Build history of the part. All positions in model axes, mm. A direction names the side the tool comes from. Coordinates: 2 decimals unless noted, no trailing zeros. Order: outer loops, then holes, each group sorted by start corner. A loop starts at its lowest first (then second) coordinate and runs counter-clockwise, first axis right, second up. Notation, with made-up numbers: (-6.75, -31) - (34.25, -31) arc R25 ccw to (34.25, -4) - close; hole circle Ø10 at (29, 86). An arc over 180 degrees is marked (long way). Write each question's results on one line, items separated by ' | '. Start each with the question number.
from build123d import *

# Parameters (mm, degrees)
EXTRUDE_1_DEPTH     = 70
CUT_EXTRUDE_1_DEPTH = 74.35529974
SKETCH_3_W          = 18.609369779
SKETCH_3_H          = 2.954088086
EXTRUDE_3_DEPTH     = 15.5
SKETCH_4_W          = 40
SKETCH_4_H          = 1
EXTRUDE_4_DEPTH     = 20
SKETCH_5_R          = 0.9
CUT_EXTRUDE_2_DEPTH = 72.281133549
SKETCH_6_W          = 3.6
SKETCH_6_H          = 3.5
SKETCH_7_R          = 1.25
CUT_EXTRUDE_3_DEPTH = 72.414284285


with BuildPart() as part:
    # ｽｹｯﾁ1 → ﾎﾞｽ - 押し出し1 (new body)
    with BuildSketch(Plane.XY):
        Polygon((-10, 0), (10, 0), (10, 3), (7.202154051, 9), (-7.202154051, 9), (-10, 3), align=None)
    extrude(amount=EXTRUDE_1_DEPTH)

    # ｽｹｯﾁ2 → ｶｯﾄ - 押し出し1 (cut, through all)
    with BuildSketch(Plane(origin=(10, 0, 0), x_dir=(0, 0, -1), z_dir=(1, 0, 0))):
        Polygon((-70, 3), (-67.202154051, 9), (-70, 9), align=None)
        Polygon((-2.797845949, 9), (0, 9), (0, 3), align=None)
    extrude(amount=-CUT_EXTRUDE_1_DEPTH, mode=Mode.SUBTRACT)

    # 面取り1
    # the kernel refuses this chamfer: 0.5 mm, written as the material it takes off along each edge
    with BuildSketch(Plane(origin=(-6.995420754, 8.697897404, 3.004579246), x_dir=(-0.8270486586180938, -0.5268881046463177, -0.19590671622030348), z_dir=(-0.41632572739388457, 0.8082980746110386, -0.41632572739387685))) as chamfer_1_piece_1:
        Polygon((-0.459173014, 0.228990916), (0.400884159, 0.228990916), (0.058288855, -0.457981831), align=None)
    extrude(amount=0.4579583, mode=Mode.SUBTRACT)
    with BuildSketch(Plane(origin=(-6.995420754, 8.697897404, 66.995420754), x_dir=(0.1959067162203077, 0.5268881046463173, -0.8270486586180933), z_dir=(-0.41632572739387774, 0.8082980746110393, 0.4163257273938825))) as chamfer_1_piece_2:
        Polygon((-0.400884159, -0.228990916), (0.459173014, -0.228990916), (-0.058288855, 0.457981831), align=None)
    extrude(amount=0.4579583, mode=Mode.SUBTRACT)
    with BuildSketch(Plane(origin=(6.995420754, 8.697897404, 3.004579246), x_dir=(0.8270486586180947, -0.5268881046463163, -0.1959067162203037), z_dir=(0.4163257273938817, 0.8082980746110384, -0.41632572739387985))) as chamfer_1_piece_3:
        Polygon((-0.459173014, -0.228990916), (0.400884159, -0.228990916), (0.058288855, 0.457981831), align=None)
    extrude(amount=0.4579583, mode=Mode.SUBTRACT)
    with BuildSketch(Plane(origin=(6.995420754, 8.697897404, 66.995420754), x_dir=(-0.19590671622030845, 0.5268881046463186, -0.8270486586180921), z_dir=(0.4163257273938828, 0.8082980746110372, 0.4163257273938814))) as chamfer_1_piece_4:
        Polygon((-0.400884159, 0.228990916), (0.459173014, 0.228990916), (-0.058288855, -0.457981831), align=None)
    extrude(amount=0.4579583, mode=Mode.SUBTRACT)
    with BuildSketch(Plane(origin=(10, -1.285841494, 70), x_dir=(0.02749587661058574, 0, -0.9996219169112968), z_dir=(0, 1, 0)), Plane(origin=(-10, 4.285841494, 70), x_dir=(-0.02749587661058574, 0, -0.9996219169112968), z_dir=(0, -1, 0))) as chamfer_1_piece_5:
        with BuildLine():
            Line((0.514336598, 0), (-0.028273577, 0.513558897))
            Line((-0.028273577, 0.513558897), (-0.038269797, 0.513283938))
            ThreePointArc((-0.038269797, 0.513283938), (-0.017064614, 0.256698915), (-0.009996219, -0.000274959))
            Line((-0.009996219, -0.000274959), (0.000274959, -0.009996219))
            ThreePointArc((0.000274959, -0.009996219), (0.257248832, -0.002927825), (0.514611556, -0.009996219))
            Line((0.514611556, -0.009996219), (0.514336598, 0))
        make_face()
    extrude(amount=5.571682988, mode=Mode.SUBTRACT)
    with BuildSketch(Plane(origin=(-7.202154051, 9, 1.505397137), x_dir=(-0.4413655645980917, -0.8973273864019796, 0), z_dir=(0, 0, 1))) as chamfer_1_piece_6:
        with BuildLine():
            Line((0.516979525, 0), (-0.237770334, 0.459056747))
            Line((-0.237770334, 0.459056747), (-0.246743608, 0.454643091))
            ThreePointArc((-0.246743608, 0.454643091), (-0.123037104, 0.227486173), (-0.008973274, -0.004413656))
            Line((-0.008973274, -0.004413656), (0.000207861, -0.009997839))
            ThreePointArc((0.000207861, -0.009997839), (0.25858594, -0.004626004), (0.517187386, -0.009997839))
            Line((0.517187386, -0.009997839), (0.516979525, 0))
        make_face()
    extrude(amount=66.989205725, mode=Mode.SUBTRACT)
    with BuildSketch(Plane(origin=(7.202154051, 9, 1.505397137), x_dir=(0.441365564598093, -0.897327386401979, 0), z_dir=(0, 0, 1))) as chamfer_1_piece_7:
        with BuildLine():
            Line((0.516979525, 0), (-0.237770334, -0.459056747))
            Line((-0.237770334, -0.459056747), (-0.246743608, -0.454643091))
            ThreePointArc((-0.246743608, -0.454643091), (-0.123037104, -0.227486173), (-0.008973274, 0.004413656))
            Line((-0.008973274, 0.004413656), (0.000207861, 0.009997839))
            ThreePointArc((0.000207861, 0.009997839), (0.25858594, 0.004626004), (0.517187386, 0.009997839))
            Line((0.517187386, 0.009997839), (0.516979525, 0))
        make_face()
    extrude(amount=66.989205725, mode=Mode.SUBTRACT)
    with BuildSketch(Plane(origin=(8.494602863, 9, 67.202154051), x_dir=(0, -0.8973273864019776, 0.4413655645980958), z_dir=(-1, 0, 0))) as chamfer_1_piece_8:
        with BuildLine():
            Line((0.516979525, 0), (-0.237770334, -0.459056747))
            Line((-0.237770334, -0.459056747), (-0.246743608, -0.454643091))
            ThreePointArc((-0.246743608, -0.454643091), (-0.123037104, -0.227486173), (-0.008973274, 0.004413656))
            Line((-0.008973274, 0.004413656), (0.000207861, 0.009997839))
            ThreePointArc((0.000207861, 0.009997839), (0.25858594, 0.004626004), (0.517187386, 0.009997839))
            Line((0.517187386, 0.009997839), (0.516979525, 0))
        make_face()
    extrude(amount=16.989205725, mode=Mode.SUBTRACT)
    with BuildSketch(Plane(origin=(6.700455124, 10.075896822, 66.700455124), x_dir=(0.18700008699946485, -0.3421923931836809, -0.920834042327616), z_dir=(0.38928162063502725, -0.83481712947899, 0.38928162063501803)), Plane(origin=(-10.501698928, 1.924103178, 70.501698928), x_dir=(-0.1870000869994657, -0.34219239318368055, -0.920834042327616), z_dir=(0.38928162063502697, 0.8348171294789901, -0.3892816206350181))) as chamfer_1_piece_9:
        with BuildLine():
            Line((0.515512576, 0), (-0.117174183, -0.502019349))
            Line((-0.117174183, -0.502019349), (-0.126965941, -0.499989208))
            ThreePointArc((-0.126965941, -0.499989208), (-0.062103739, -0.250280562), (-0.009791758, 0.002030141))
            Line((-0.009791758, 0.002030141), (0.000248629, 0.009996909))
            ThreePointArc((0.000248629, 0.009996909), (0.257845581, 0.003590326), (0.515761205, 0.009996909))
            Line((0.515761205, 0.009996909), (0.515512576, 0))
        make_face()
    extrude(amount=9.764765667, mode=Mode.SUBTRACT)
    with BuildSketch(Plane(origin=(6.700455124, 10.075896822, 3.299544876), x_dir=(0.18700008699946544, -0.34219239318368183, 0.9208340423276157), z_dir=(0.38928162063502697, -0.8348171294789896, -0.38928162063501903)), Plane(origin=(-10.501698928, 1.924103178, -0.501698928), x_dir=(-0.18700008699946621, -0.3421923931836814, 0.9208340423276155), z_dir=(0.38928162063502675, 0.8348171294789897, 0.3892816206350191))) as chamfer_1_piece_10:
        with BuildLine():
            Line((0.515512576, 0), (-0.117174183, 0.502019349))
            Line((-0.117174183, 0.502019349), (-0.126965941, 0.499989208))
            ThreePointArc((-0.126965941, 0.499989208), (-0.062103739, 0.250280562), (-0.009791758, -0.002030141))
            Line((-0.009791758, -0.002030141), (0.000248629, -0.009996909))
            ThreePointArc((0.000248629, -0.009996909), (0.257845581, -0.003590326), (0.515761205, -0.009996909))
            Line((0.515761205, -0.009996909), (0.515512576, 0))
        make_face()
    extrude(amount=9.764765667, mode=Mode.SUBTRACT)
    with BuildSketch(Plane(origin=(8.494602863, 9, 2.797845949), x_dir=(0, -0.8973273864019827, -0.44136556459808546), z_dir=(-1, 0, 0))) as chamfer_1_piece_11:
        with BuildLine():
            Line((0.516979525, 0), (-0.237770334, 0.459056747))
            Line((-0.237770334, 0.459056747), (-0.246743608, 0.454643091))
            ThreePointArc((-0.246743608, 0.454643091), (-0.123037104, 0.227486173), (-0.008973274, -0.004413656))
            Line((-0.008973274, -0.004413656), (0.000207861, -0.009997839))
            ThreePointArc((0.000207861, -0.009997839), (0.25858594, -0.004626004), (0.517187386, -0.009997839))
            Line((0.517187386, -0.009997839), (0.516979525, 0))
        make_face()
    extrude(amount=16.989205725, mode=Mode.SUBTRACT)
    with BuildSketch(Plane(origin=(10, -1.285841494, 0), x_dir=(0.02749587661058563, 0, 0.9996219169112968), z_dir=(0, 1, 0)), Plane(origin=(-10, 4.285841494, 0), x_dir=(-0.02749587661058563, 0, 0.9996219169112968), z_dir=(0, -1, 0))) as chamfer_1_piece_12:
        with BuildLine():
            Line((0.514336598, 0), (-0.028273577, -0.513558897))
            Line((-0.028273577, -0.513558897), (-0.038269797, -0.513283938))
            ThreePointArc((-0.038269797, -0.513283938), (-0.017064614, -0.256698915), (-0.009996219, 0.000274959))
            Line((-0.009996219, 0.000274959), (0.000274959, 0.009996219))
            ThreePointArc((0.000274959, 0.009996219), (0.257248832, 0.002927825), (0.514611556, 0.009996219))
            Line((0.514611556, 0.009996219), (0.514336598, 0))
        make_face()
    extrude(amount=5.571682988, mode=Mode.SUBTRACT)

    # ｽｹｯﾁ3 → ﾎﾞｽ - 押し出し3 (add)
    with BuildSketch(Plane.XY.offset(70)):
        with Locations((-0.19531511, 1.477044043)):
            Rectangle(SKETCH_3_W, SKETCH_3_H)
    extrude(amount=-EXTRUDE_3_DEPTH)

    # ｽｹｯﾁ4 → ﾎﾞｽ - 押し出し4 (add)
    with BuildSketch(Plane.ZY.offset(10)):
        with Locations((35, -0.5)):
            Rectangle(SKETCH_4_W, SKETCH_4_H)
    extrude(amount=-EXTRUDE_4_DEPTH)

    # ｽｹｯﾁ5 → ｶｯﾄ - 押し出し2 (cut, through all)
    with BuildSketch(Plane(origin=(0, 0, 0), x_dir=(-1, 0, 0), z_dir=(0, 0, -1))):
        with Locations((0, 1.78)):
            Circle(SKETCH_5_R)
    extrude(amount=-CUT_EXTRUDE_2_DEPTH, mode=Mode.SUBTRACT)

    # ｽｹｯﾁ6 → ｶｯﾄ - 回転1 (revolve, cut)
    with BuildSketch(Plane(origin=(0, 1.78, 0), x_dir=(-1, 0, 0), z_dir=(0, -1, 0))):
        with Locations((1.8, -62)):
            Rectangle(SKETCH_6_W, SKETCH_6_H)
        with Locations((1.8, -8)):
            Rectangle(SKETCH_6_W, SKETCH_6_H)
    revolve(axis=Axis((0, 1.78, 70), (0, 0, -1)), mode=Mode.SUBTRACT)

    # ｽｹｯﾁ7 → ｶｯﾄ - 押し出し3 (cut, through all)
    with BuildSketch(Plane(origin=(0, 9, 0), x_dir=(1, 0, 0), z_dir=(0, 1, 0))):
        with Locations(Location((-5, -35, 0), (0, 0, 180))):
            Circle(SKETCH_7_R)
        with Locations(Location((5, -35, 0), (0, 0, 180))):
            Circle(SKETCH_7_R)
    extrude(amount=-CUT_EXTRUDE_3_DEPTH, mode=Mode.SUBTRACT)


solid = part.part
Item 1: Slice it at B-B (z = 35). Write the cut outline in (x, y).
Item 2: Pull direction Y, two halves, no side cores. Call faces 4 (the flat face through (0, 0, 64)), 5 (the flat face through (0, 9, 35)), 6 (the cylindrical face through (0.12, 2.67, 3.08)), 7 (the cylindrical face through (0.12, 2.67, 34.65)): released by +Y, released by -Y, zero draft, split by the parting line, or undercut.
Item 3: Probe probe 1 along X at (y, z) = (1.78, 62.55); probe 2 along Z at (x, y) = (-0.25, 4.5); probe 3 along Y at (x, z) = (0, 61.4). List the from-to ranges inside material, lowest first.
Item 4: Slice it at D-D (z = 52). Write the cut outline in (x, y).
Item 5: Which spindle directions (+Z, -Z, +X, -X, +Y, -Y) get a long thin tool onto all of the face, cutting with end or side? Do faces 1 (the flat face through (0, 0, 6)), 2 (the flat face through (-0.1, 0.5, 0)), 3 (the flat face through (0, 3, 6.25)). Say none if no direction does.
Item 6: Slice it at A-A (y = 1.78). Count the separate pieces of the cut face and the enclosed holes in it, then the cut area to 3 significant figures.
Item 7: Flat gauge pins, fed straight in: P1, Ø1.5, axis at y = 5.5, z = 9.5, coming from the -X side; P2, Ø4.5, axis at x = -2.5, z = 65.5, coming from the -Y side; P3, Ø4, axis at y = 5.5, z = 18.5, coming from the +X side. Where does each tip first touch, or does it go through?
Resolved:
1) outline: (-10, -1) - (-6.25, -1) - (-6.25, 9) - (-6.7, 9) - (-7.41, 8.55) - (-10, 3) - close; (-3.75, -1) - (3.75, -1) - (3.75, 9) - (-3.75, 9) - close; (6.25, -1) - (10, -1) - (10, 3) - (7.41, 8.55) - (6.7, 9) - (6.25, 9) - close; hole circle Ø1.8 at (0, 1.78)
2) face 4: released by -Y | face 5: released by +Y | face 6: undercut | face 7: undercut
3) probe 1: -10 to -3.6, 3.6 to 10 | probe 2: 0.7 to 6.25, 9.75 to 60.25, 63.75 to 69.3 | probe 3: 5.38 to 9
4) outline: (-10, -1) - (10, -1) - (10, 3) - (7.41, 8.55) - (6.7, 9) - (-6.7, 9) - (-7.41, 8.55) - (-10, 3) - close; hole circle Ø1.8 at (0, 1.78)
5) face 1: -Z, +X, -X, -Y | face 2: -Z, +X, -X, +Y, -Y | face 3: none
6) separate pieces: 2 | enclosed holes: 2 | area: 1,230 mm^2
7) P1: x = -9.18 | P2: y = 0 | P3: x = 9.77
